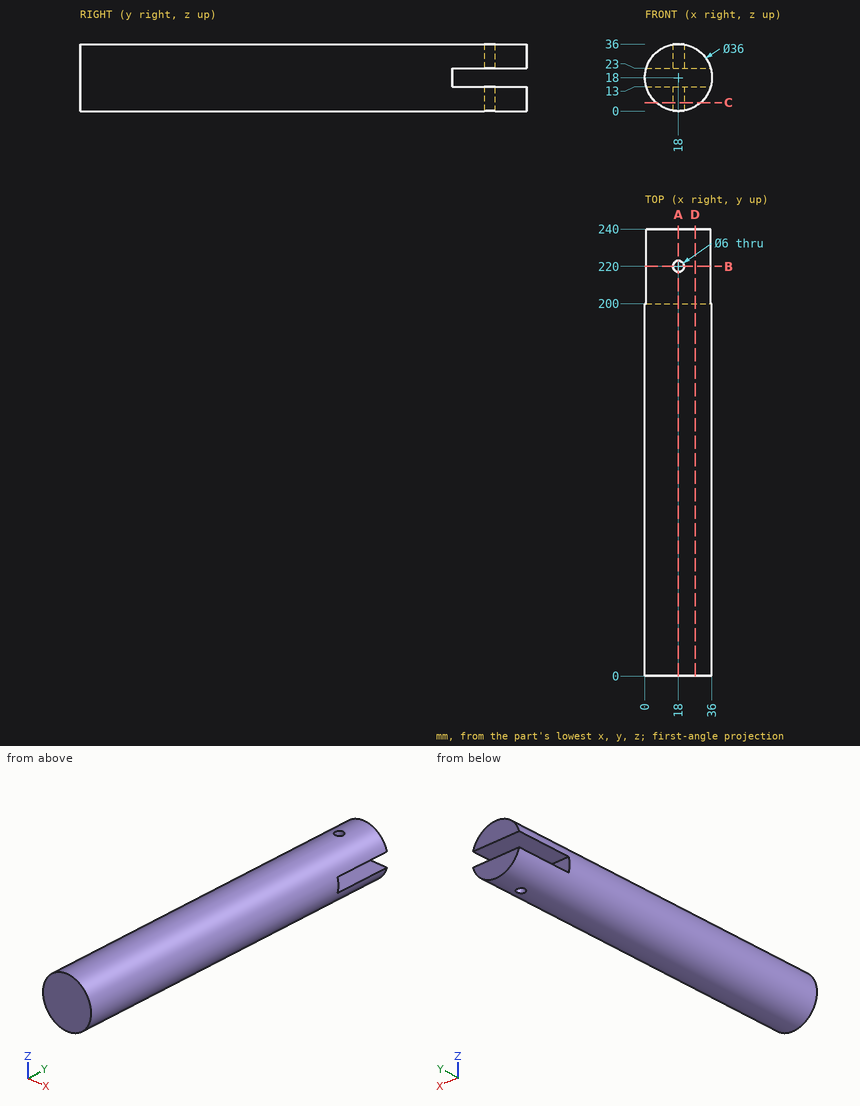
Geometry: see drawing. Coordinates: mm, zero at the bounding-box minimum. Give positions to 0.01 mm unless a question says otherwise; leave off trailing zeros. Write each loop counter-clockwise with the first axis right and the second up, starting at its lowest first coordinate (ties: lowest second). Pieces come first, ordered by that corner, then holes. Notation, with made-up numbers: M 41.25,-25 L 78.25,-25 A8 ccw 78.25,-10 Z; hole C 22.5,86.5 d4. An arc over 180 degrees is marked long. Return JSON: item names as keys, results as strings. Group by question number.
1) Cut plane A-A, the plane x = 18. Output: boundary loops of the cut face in (y, z), then the cut area to 3 significant figures.
2) Cut plane B-B, the plane y = 220. Output: boundary loops of the cut face in (x, z), then the cut area to 3 significant figures.
3) Cut plane C-C, the plane z = 4.5. Output: boundary loops of the cut face in (x, y), then the cut area to 3 significant figures.
4) Ray query, L1, parallel to Y at x = 32, z = 15; L2, parallel to Z at x = 17.5, y = 210; L3, parallel to Y at x = 16.5, z = 34. Return the intervals inside material, ascending.
5) First-contact query: pin 1 Ø1.5 at (x, y) = (8.5, 136) entering from +Z; pin 2 Ø3 at (x, z) = (15.5, 20) entering from +Y; pin 3 Ø5.5 at (x, y) = (18, 220) entering from -Z; pin 4 Ø10.5 at (x, y) = (11, 211.5) entering from +Z. Flat tips, straight axial feed; report the tip coordinate or a pass-through.
6) Cut plane D-D, the plane x = 27. Output: boundary loops of the cut face in (y, z), then the cut area to 3 significant figures.
Data:
{
 "1": {"outline": "M 0,0 L 217,0 L 217,13 L 200,13 L 200,23 L 217,23 L 217,36 L 0,36 Z; M 223,0 L 240,0 L 240,13 L 223,13 Z; M 223,23 L 240,23 L 240,36 L 223,36 Z", "area": "8,080 mm²"},
 "2": {"outline": "M 0.71,13 A18 ccw 15,0.25 L 15,13 Z; M 0.71,23 L 15,23 L 15,35.75 A18 ccw Z; M 21,0.25 A18 ccw 35.29,13 L 21,13 Z; M 21,23 L 35.29,23 A18 ccw 21,35.75 Z", "area": "508 mm²"},
 "3": {"outline": "M 6.09,0 L 29.91,0 L 29.91,240 L 6.09,240 Z; hole C 18,220 d6", "area": "5,690 mm²"},
 "4": {"L1": "y = 0 to 200", "L2": "z = 0.01 to 13, 23 to 35.99", "L3": "y = 0 to 217.4, 222.6 to 240"},
 "5": {"pin 1": "stops at z = 33.73", "pin 2": "stops at y = 200", "pin 3": "passes through", "pin 4": "stops at z = 35.91"},
 "6": {"outline": "M 0,2.41 L 240,2.41 L 240,13 L 200,13 L 200,23 L 240,23 L 240,33.59 L 0,33.59 Z", "area": "7,080 mm²"}
}
